Can you work these out from the model? Positions are in its coordinate system, mm. Round coordinates to 2 decimals unless told otherwise and drop trailing zeros. Loops run counter-clockwise (first coordinate to the right, second up) from the corner with the lowest first, then second, coordinate; pieces in that order, holes last. Notation, with made-up numbers: (66, -24) - (117, -24) arc R17 ccw to (117, -7) - close; hole circle Ø7 at (-35, -1). An arc over 180 degrees is marked (long way). Answer as CSV lines item,"result".
```python
from build123d import *

# Parameters (mm, degrees)
SKETCH1_R           = 7.5
SKETCH1_R_2         = 12.5
SKETCH1_R_3         = 3
BOSS_EXTRUDE1_DEPTH = 3.5


with BuildPart() as part:
    # Sketch1 → Boss-Extrude1 (new body, symmetric)
    with BuildSketch(Plane.XY):
        with BuildLine():
            Line((-38, -18), (38, -18))
            ThreePointArc((38, -18), (53.238850443, -9.580054133), (54.221001351, 7.802506979))
            Line((54.221001351, 7.802506979), (16.221001351, 86.802506979))
            ThreePointArc((16.221001351, 86.802506979), (0, 97), (-16.221001351, 86.802506979))
            Line((-16.221001351, 86.802506979), (-54.221001351, 7.802506979))
            ThreePointArc((-54.221001351, 7.802506979), (-53.238850443, -9.580054133), (-38, -18))
        make_face()
        with Locations((-38, 0)):
            Circle(SKETCH1_R, mode=Mode.SUBTRACT)
        with Locations((38, 0)):
            Circle(SKETCH1_R, mode=Mode.SUBTRACT)
        with Locations((0, 14)):
            Circle(SKETCH1_R_2, mode=Mode.SUBTRACT)
        with Locations((-15.155444566, 22.75)):
            Circle(SKETCH1_R_3, mode=Mode.SUBTRACT)
        with Locations((0, -3.5)):
            Circle(SKETCH1_R_3, mode=Mode.SUBTRACT)
        with Locations((15.155444566, 22.75)):
            Circle(SKETCH1_R_3, mode=Mode.SUBTRACT)
        with Locations((0, 79)):
            Circle(SKETCH1_R, mode=Mode.SUBTRACT)
    extrude(amount=BOSS_EXTRUDE1_DEPTH, both=True)


solid = part.part
```
Q1. We'd pull the mould along Y, two halves only. Please class faces 1 (the flat face through (-1, 28, -3.5)), 2 (the cylindrical face through (0, 97, 0)), 3 (the cylindrical face through (-2.71, 1.797, -0.049)), 4 (the cylindrical face through (12.775, 20.925, -0.049)): pulls with the +Y half, pulls with the -Y half, needs draft (parallel to the pull), parting line crosses it, or undercut.
Checks:
face 1,"needs draft"
face 2,"pulls with the +Y half"
face 3,"undercut"
face 4,"undercut"
Q2. Imagine slicing it at B-B (y = 22.75). Write out the boundary of the cut face in (x, z), then the cut area to 3 significant figures.
Checks:
outline,"(-47.03, -3.5) - (-18.16, -3.5) - (-18.16, 3.5) - (-47.03, 3.5) - close; (-12.16, -3.5) - (-8.93, -3.5) - (-8.93, 3.5) - (-12.16, 3.5) - close; (8.93, -3.5) - (12.16, -3.5) - (12.16, 3.5) - (8.93, 3.5) - close; (18.16, -3.5) - (47.03, -3.5) - (47.03, 3.5) - (18.16, 3.5) - close"
area,"449 mm²"
Q3. Imagine slicing it at A-A (x = 0). Write out the boundary of the cut face in (y, z).
Checks:
outline,"(-18, -3.5) - (-6.5, -3.5) - (-6.5, 3.5) - (-18, 3.5) - close; (-0.5, -3.5) - (1.5, -3.5) - (1.5, 3.5) - (-0.5, 3.5) - close; (26.5, -3.5) - (71.5, -3.5) - (71.5, 3.5) - (26.5, 3.5) - close; (86.5, -3.5) - (97, -3.5) - (97, 3.5) - (86.5, 3.5) - close"
Q4. Imagine slicing it at D-D (y = 83). Write out the boundary of the cut face in (x, z).
Checks:
outline,"(-18.05, -3.5) - (-6.34, -3.5) - (-6.34, 3.5) - (-18.05, 3.5) - close; (6.34, -3.5) - (18.05, -3.5) - (18.05, 3.5) - (6.34, 3.5) - close"
Q5. I'm going to push flat-ended pins straight in: pin 1 Ø1 at (y, z) = (5, 0.5) entering from -X; pin 2 Ø2 at (y, z) = (7, 1.5) entering from +X; pin 3 Ø2 at (x, z) = (6.5, -2) entering from +Y. Where does each tip first touch, or does it pass through?
Checks:
pin 1,"x = -55.43"
pin 2,"x = 54.97"
pin 3,"y = 96.14"
Q6. Imagine slicing it at C-C (z = 0.5). Write out the boundary of the cut face in (x, y).
Checks:
outline,"(-54.22, 7.8) arc R18 ccw to (-38, -18) - (38, -18) arc R18 ccw to (54.22, 7.8) - (16.22, 86.8) arc R18 ccw to (-16.22, 86.8) - close; hole circle Ø15 at (-38, 0); hole circle Ø6 at (-15.16, 22.75); hole circle Ø25 at (0, 14); hole circle Ø15 at (0, 79); hole circle Ø6 at (0, -3.5); hole circle Ø6 at (15.16, 22.75); hole circle Ø15 at (38, 0)"
Q7. If I drill on line 1 along Y through (x, z) = (0, 1.25); line 2 along X through (y, z) = (-3, 1.25); line 3 along Y through (x, z) = (-4.5, -1), over which ranges is the centre line in solid material (lowest first)? Write a range as [from, to].
Checks:
line 1,"[-18, -6.5], [-0.5, 1.5], [26.5, 71.5], [86.5, 97]"
line 2,"[-55.75, -44.87], [-31.13, -2.96], [2.96, 31.13], [44.87, 55.75]"
line 3,"[-18, 2.34], [25.66, 73], [85, 96.43]"
